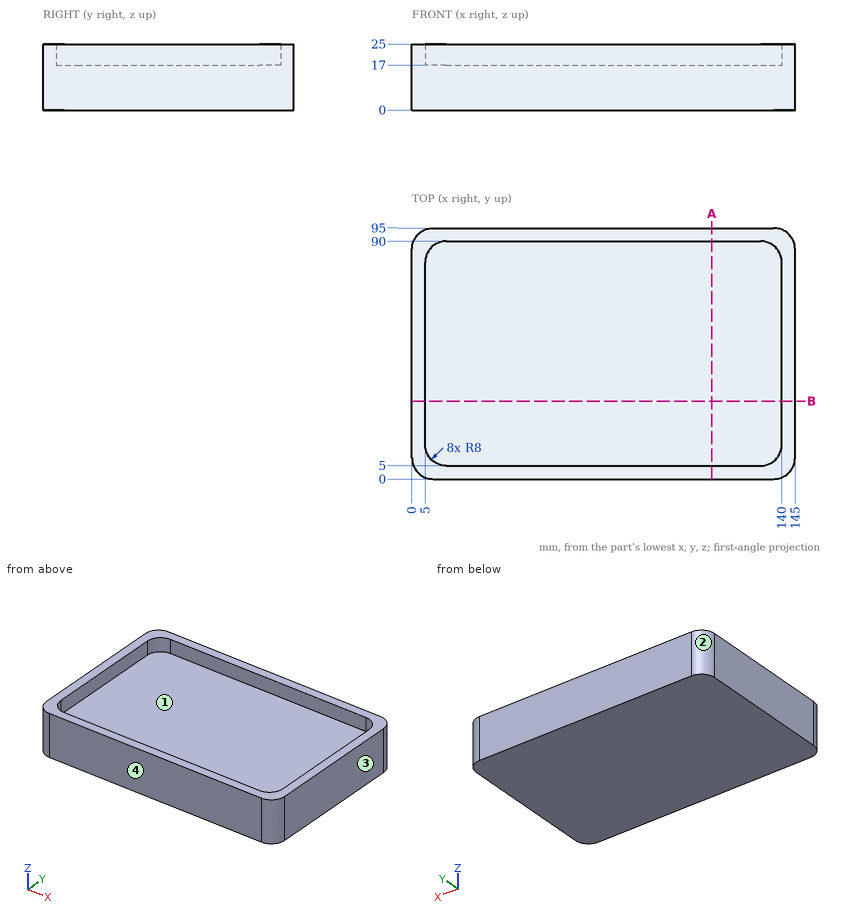
Input: dimensioned drawing with shaded views. Units: mm. Origin: part minimum x, y, z. Round coordinates to 2 decimals unless told otherwise and drop trailing zeros. Loops run counter-clockwise (first coordinate to the right, second up) from the corner with the lowest first, then second, coordinate; pieces in that order, holes last.
1) Material intervals for line 1 (X direction, y = 70, z = 17.5); line 2 (Y direction, x = 34, z = 19.75); line 3 (Z direction, x = 22.5, y = 31), sorted ascending.
Ans:
line 1: x = 0 to 5, 140 to 145
line 2: y = 0 to 5, 90 to 95
line 3: z = 0 to 17
2) Section query A-A on x = 113.5. Return the cut outline in (y, z), plus the area to 4 significant figures.
Ans:
outline: (0, 0) - (95, 0) - (95, 25) - (90, 25) - (90, 17) - (5, 17) - (5, 25) - (0, 25) - close
area: 1,695 mm2
3) Pull-direction query (Y, two-part tool) for the marked faces 1, 2, 3 and 4; classes: released by +Y, released by -Y, zero draft, split by the parting line, or undercut.
Ans:
face 1: undercut
face 2: released by +Y
face 3: zero draft
face 4: released by -Y
4) Pin query (flat end, axial travel): pin 1 (9 mm diameter, centred on y = 53.5, z = 21.5, fed in from -X); pin 2 (10 mm diameter, centred on x = 65, y = 49.5, fed in from +Z). Return the tip coordinate at first contact, or that it passes through.
Ans:
pin 1: stops at x = 0
pin 2: stops at z = 17
5) Section query B-B on y = 29.5. Return the cut outline in (x, z).
Ans:
outline: (0, 0) - (145, 0) - (145, 25) - (140, 25) - (140, 17) - (5, 17) - (5, 25) - (0, 25) - close
